```python
from build123d import *

# Parameters (mm, degrees)
CROQUIS1_W              = 34
CROQUIS1_H              = 22
SALIENTE_EXTRUIR1_DEPTH = 11
CROQUIS2_W              = 14
CROQUIS2_H              = 22
SALIENTE_EXTRUIR2_DEPTH = 3
CHAFL_N1_SIZE           = 2
CHAFL_N1_SIZE2          = 2.383507185
CROQUIS3_R              = 0.5
SALIENTE_EXTRUIR3_DEPTH = 150


with BuildPart() as part:
    # Croquis1 → Saliente-Extruir1 (new body)
    with BuildSketch(Plane.XY):
        Rectangle(CROQUIS1_W, CROQUIS1_H)
    extrude(amount=SALIENTE_EXTRUIR1_DEPTH)

    # Croquis2 → Saliente-Extruir2 (add)
    with BuildSketch(Plane.XY.offset(11)):
        with Locations((-10, 0)):
            Rectangle(CROQUIS2_W, CROQUIS2_H)
    extrude(amount=SALIENTE_EXTRUIR2_DEPTH)

    # Chaflán1
    chafl_n1_edges = [part.edges().sort_by_distance(p)[0] for p in [
        (-3, 0, 14),
    ]]
    chafl_n1_side = [part.faces().sort_by_distance(p)[0] for p in [
        (-3, 0, 12.5),
    ]]
    chamfer(chafl_n1_edges, length=CHAFL_N1_SIZE, length2=CHAFL_N1_SIZE2, reference=chafl_n1_side[0])

    # Croquis3 → Saliente-Extruir3 (add)
    with BuildSketch(Plane(origin=(17, 0, 0), x_dir=(0, 0, -1), z_dir=(1, 0, 0))):
        with Locations((-5.5, 0)):
            Circle(CROQUIS3_R)
    extrude(amount=SALIENTE_EXTRUIR3_DEPTH)


solid = part.part
```
Geometry check sheet. Reference: the model listing, model coordinates, mm. A direction names the side the tool comes from. Coordinates: 2 decimals unless noted, no trailing zeros. Loops run counter-clockwise (first coordinate to the right, second up) from the corner with the lowest first, then second, coordinate; pieces in that order, holes last.
Item 1: Sectioned sample at B-B, the plane x = 22. Record the boundary of the cut face in (y, z).
Item 2: Thickness scan on line 1 (X direction, y = 7.75, z = 2.25); line 2 (X direction, y = -9.75, z = 11.5); line 3 (Z direction, x = 15, y = 6.25). Record the ranges inside material, lowest first.
Item 3: Access from +Z, -Z, +X, -X, +Y, -Y to the whole of each face (thin tool, end or side, straight path). Record for faces 1 (the face through (7, 0, 11)), 2 (the face through (0, -11, 5)).
Item 4: Sectioned sample at C-C, the plane z = 8. Record the boundary of the cut face in (x, y), then the cut area to 3 significant figures.
Item 5: Go/stop test with flat-tipped pins: pin 1 Ø6 at (x, y) = (8, 2) entering from +Z; pin 2 Ø6 at (x, z) = (76.5, 7.5) entering from -Y; pin 3 Ø1.1 at (y, z) = (-3.5, 11.5) entering from +X; pin 4 Ø4 at (x, z) = (108, 9) entering from +Y. Record where each tip stops, or that it passes through.
Item 6: Sectioned sample at A-A, the plane y = -2.25. Record the boundary of the cut face in (x, z), then the cut area to 3 significant figures.
Check result:
1. outline: circle Ø1 at (0, 5.5)
2. line 1: x = -17 to 17
2. line 2: x = -17 to -3
2. line 3: z = 0 to 11
3. face 1: +Z, +X, +Y, -Y
3. face 2: +Z, -Z, +X, -X, -Y
4. outline: (-17, -11) - (17, -11) - (17, 11) - (-17, 11) - close
4. area: 748 mm2
5. pin 1: stops at z = 11
5. pin 2: stops at y = -0.5
5. pin 3: stops at x = 17
5. pin 4: passes through
6. outline: (-17, 0) - (17, 0) - (17, 11) - (-3, 11) - (-3, 12) - (-5.38, 14) - (-17, 14) - close
6. area: 414 mm2
